```python
from build123d import *

# Parameters (mm, degrees)
SKETCH1_R           = 1.6
BOSS_EXTRUDE1_DEPTH = 4.1
CUT_EXTRUDE1_DEPTH  = 2
FILLET2_R           = 10
CUT_EXTRUDE4_DEPTH  = 52.043216983
SKETCH7_W           = 35
SKETCH7_H           = 20
CUT_EXTRUDE5_DEPTH  = 52.043216983


with BuildPart() as part:
    # Sketch1 → Boss-Extrude1 (new body)
    with BuildSketch(Plane(origin=(0, 0, 0), x_dir=(1, 0, 0), z_dir=(0, 1, 0))):
        Polygon((15.934040652, 35), (-15.934040652, 35), (-23.334523779, 36.062445841), (-36.062445841, 23.334523779), (-35, 15.934040652), (-35, -15.934040652), (-36.062445841, -23.334523779), (-23.334523779, -36.062445841), (-15.934040652, -35), (15.934040652, -35), (23.334523779, -36.062445841), (36.062445841, -23.334523779), (35, -15.934040652), (35, 15.934040652), (36.062445841, 23.334523779), (23.334523779, 36.062445841), align=None)
        with Locations(Location((22.627416998, 31.112698372, 0), (0, 0, 270))):
            Circle(SKETCH1_R, mode=Mode.SUBTRACT)
        with Locations(Location((31.112698372, 22.627416998, 0), (0, 0, 270))):
            Circle(SKETCH1_R, mode=Mode.SUBTRACT)
        with Locations(Location((22.627416998, -31.112698372, 0), (0, 0, 270))):
            Circle(SKETCH1_R, mode=Mode.SUBTRACT)
        with Locations(Location((31.112698372, -22.627416998, 0), (0, 0, 270))):
            Circle(SKETCH1_R, mode=Mode.SUBTRACT)
        with Locations(Location((-31.112698372, -22.627416998, 0), (0, 0, 270))):
            Circle(SKETCH1_R, mode=Mode.SUBTRACT)
        with Locations(Location((-22.627416998, -31.112698372, 0), (0, 0, 270))):
            Circle(SKETCH1_R, mode=Mode.SUBTRACT)
        with Locations(Location((-22.627416998, 31.112698372, 0), (0, 0, 270))):
            Circle(SKETCH1_R, mode=Mode.SUBTRACT)
        with Locations(Location((-31.112698372, 22.627416998, 0), (0, 0, 270))):
            Circle(SKETCH1_R, mode=Mode.SUBTRACT)
    extrude(amount=BOSS_EXTRUDE1_DEPTH)

    # Sketch2 → Cut-Extrude1 (cut)
    with BuildSketch(Plane(origin=(0, 4.1, 0), x_dir=(1, 0, 0), z_dir=(0, 1, 0))):
        Polygon((-17.669047558, 29), (17.669047558, 29), (29, 17.669047558), (29, -17.669047558), (17.669047558, -29), (-17.669047558, -29), (-29, -17.669047558), (-29, 17.669047558), align=None)
    extrude(amount=-CUT_EXTRUDE1_DEPTH, mode=Mode.SUBTRACT)

    # Fillet2
    fillet2_edges = [part.edges().sort_by_distance(p)[0] for p in [
        (-15.934040652, 2.05, -35),
        (15.934040652, 2.05, -35),
        (35, 2.05, -15.934040652),
        (35, 2.05, 15.934040652),
        (15.934040652, 2.05, 35),
        (-15.934040652, 2.05, 35),
        (-35, 2.05, 15.934040652),
        (-35, 2.05, -15.934040652),
    ]]
    fillet(fillet2_edges, radius=FILLET2_R)

    # Sketch6 → Cut-Extrude4 (cut, through all)
    with BuildSketch(Plane(origin=(0, 2.1, 0), x_dir=(1, 0, 0), z_dir=(0, 1, 0))):
        with BuildLine():
            Line((-1.5, 19.7), (-1.5, 18.3))
            ThreePointArc((-1.5, 18.3), (-1.734314575, 17.734314575), (-2.3, 17.5))
            Line((-2.3, 17.5), (-6.7, 17.5))
            ThreePointArc((-6.7, 17.5), (-7.265685425, 17.734314575), (-7.5, 18.3))
            Line((-7.5, 18.3), (-7.5, 26.7))
            ThreePointArc((-7.5, 26.7), (-7.265685425, 27.265685425), (-6.7, 27.5))
            Line((-6.7, 27.5), (6.7, 27.5))
            ThreePointArc((6.7, 27.5), (7.265685425, 27.265685425), (7.5, 26.7))
            Line((7.5, 26.7), (7.5, 18.3))
            ThreePointArc((7.5, 18.3), (7.265685425, 17.734314575), (6.7, 17.5))
            Line((6.7, 17.5), (2.3, 17.5))
            ThreePointArc((2.3, 17.5), (1.734314575, 17.734314575), (1.5, 18.3))
            Line((1.5, 18.3), (1.5, 19.7))
            ThreePointArc((1.5, 19.7), (1.734314575, 20.265685425), (2.3, 20.5))
            Line((2.3, 20.5), (4.2, 20.5))
            ThreePointArc((4.2, 20.5), (4.765685425, 20.734314575), (5, 21.3))
            Line((5, 21.3), (5, 23.7))
            ThreePointArc((5, 23.7), (4.765685425, 24.265685425), (4.2, 24.5))
            Line((4.2, 24.5), (-4.2, 24.5))
            ThreePointArc((-4.2, 24.5), (-4.765685425, 24.265685425), (-5, 23.7))
            Line((-5, 23.7), (-5, 21.3))
            ThreePointArc((-5, 21.3), (-4.765685425, 20.734314575), (-4.2, 20.5))
            Line((-4.2, 20.5), (-2.3, 20.5))
            ThreePointArc((-2.3, 20.5), (-1.734314575, 20.265685425), (-1.5, 19.7))
        make_face()
        with BuildLine():
            Line((2.3, -17.5), (6.7, -17.5))
            ThreePointArc((6.7, -17.5), (7.265685425, -17.734314575), (7.5, -18.3))
            Line((7.5, -18.3), (7.5, -26.7))
            ThreePointArc((7.5, -26.7), (7.265685425, -27.265685425), (6.7, -27.5))
            Line((6.7, -27.5), (-6.7, -27.5))
            ThreePointArc((-6.7, -27.5), (-7.265685425, -27.265685425), (-7.5, -26.7))
            Line((-7.5, -26.7), (-7.5, -18.3))
            ThreePointArc((-7.5, -18.3), (-7.265685425, -17.734314575), (-6.7, -17.5))
            Line((-6.7, -17.5), (-2.3, -17.5))
            ThreePointArc((-2.3, -17.5), (-1.734314575, -17.734314575), (-1.5, -18.3))
            Line((-1.5, -18.3), (-1.5, -19.7))
            ThreePointArc((-1.5, -19.7), (-1.734314575, -20.265685425), (-2.3, -20.5))
            Line((-2.3, -20.5), (-4.2, -20.5))
            ThreePointArc((-4.2, -20.5), (-4.765685425, -20.734314575), (-5, -21.3))
            Line((-5, -21.3), (-5, -23.7))
            ThreePointArc((-5, -23.7), (-4.765685425, -24.265685425), (-4.2, -24.5))
            Line((-4.2, -24.5), (4.2, -24.5))
            ThreePointArc((4.2, -24.5), (4.765685425, -24.265685425), (5, -23.7))
            Line((5, -23.7), (5, -21.3))
            ThreePointArc((5, -21.3), (4.765685425, -20.734314575), (4.2, -20.5))
            Line((4.2, -20.5), (2.3, -20.5))
            ThreePointArc((2.3, -20.5), (1.734314575, -20.265685425), (1.5, -19.7))
            Line((1.5, -19.7), (1.5, -18.3))
            ThreePointArc((1.5, -18.3), (1.734314575, -17.734314575), (2.3, -17.5))
        make_face()
    extrude(amount=-CUT_EXTRUDE4_DEPTH, mode=Mode.SUBTRACT)

    # Sketch7 → Cut-Extrude5 (cut, through all)
    with BuildSketch(Plane(origin=(0, 2.1, 0), x_dir=(1, 0, 0), z_dir=(0, 1, 0))):
        Rectangle(SKETCH7_W, SKETCH7_H)
    extrude(amount=-CUT_EXTRUDE5_DEPTH, mode=Mode.SUBTRACT)


solid = part.part
```
CAD build for the part. Positions are in the model's coordinates, mm. A direction names the side the tool comes from. Coordinates: 2 decimals unless noted, no trailing zeros. Order: outer loops, then holes, each group sorted by start corner. A loop starts at its lowest first (then second) coordinate and runs counter-clockwise, first axis right, second up.
(1) Which spindle directions (+Z, -Z, +X, -X, +Y, -Y) get a long thin tool onto all of the face, cutting with end or side? Do faces 1 (the face through (-19.941, 2.021, -35.575)), 2 (the face through (7.5, 1, -23)), 3 (the face through (19.941, 2.021, 35.575)), 4 (the face through (35.59, 2.02, 20.03)). Say none if no direction does.
Solution:
face 1: -Z, +Y, -Y
face 2: +Y, -Y
face 3: +Z, +Y, -Y
face 4: +X, +Y, -Y
(2) Drill centre lines: L1, parallel to X at y = 1.7, z = 4; L2, parallel to Z at x = 2.5, y = 3.4; L3, parallel to X at y = 3.95, z = 30. Where is each one in solid material? Low to high.
Solution:
L1: x = -35 to -17.5, 17.5 to 35
L2: z = -35 to -29, 29 to 35
L3: x = -29.4 to -23.78, -21.48 to 21.48, 23.78 to 29.4
(3) Pin check, flat tips, straight feed: pin 1 Ø1.7 at (x, y) = (1, 1.5) entering from -Z; pin 2 Ø1.9 at (x, z) = (-22.63, 31.11) entering from +Y; pin 3 Ø2 at (y, z) = (3, 4.5) entering from -X; pin 4 Ø0.6 at (x, y) = (-1, 1) entering from +Z. Stop position of each tip, or through.
Solution:
pin 1: stops at z = -35
pin 2: passes through
pin 3: stops at x = -35
pin 4: stops at z = 35
(4) Saw through at C-C, the plane y = 1.25. Count the separate pieces of the cut face and the enclosed holes in it, and give its area (3 significant figures).
Solution:
separate pieces: 1
enclosed holes: 11
area: 3,750 mm2
(5) Saw through at B-B, the plane x = -20. Write the cut outline in (y, z), and give its area (3 significant figures).
Solution:
outline: (0, -35.58) - (4.1, -35.58) - (4.1, -26.67) - (2.1, -26.67) - (2.1, 26.67) - (4.1, 26.67) - (4.1, 35.58) - (0, 35.58) - close
area: 185 mm2
(6) Mould opens along X. For faces 5 (the face through (35, 2, 0)), 6 (the face through (-29.526, 2.021, -22.836)), 7 (the face through (-1, 0, -17)) say: released by +X, released by -X, zero draft, split by the parting line, or undercut.
Solution:
face 5: released by +X
face 6: undercut
face 7: zero draft
(7) Saw through at A-A, the plane z = -6. Write the cut outline in (x, y), and give its area (3 significant figures).
Solution:
outline: (-35, 0) - (-17.5, 0) - (-17.5, 2.1) - (-29, 2.1) - (-29, 4.1) - (-35, 4.1) - close; (17.5, 0) - (35, 0) - (35, 4.1) - (29, 4.1) - (29, 2.1) - (17.5, 2.1) - close
area: 97.5 mm2
